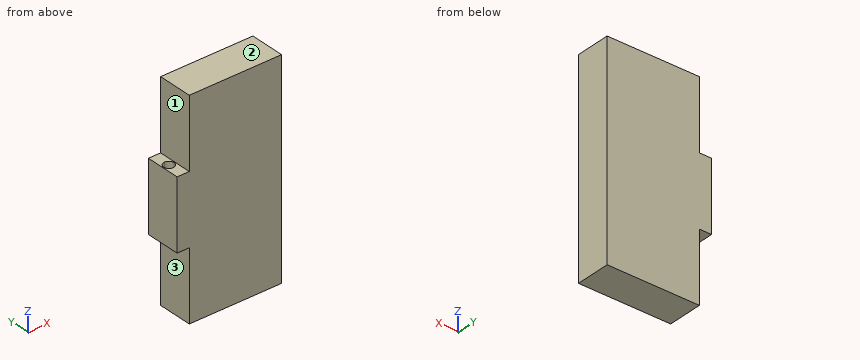
```python
from build123d import *

# Parameters (mm, degrees)
F1_DEPTH = 25.4
F3_DEPTH = 101.601


with BuildPart() as f1:
    # F0 (on Front) → F1 (new body)
    with BuildSketch(Plane.XZ):
        Polygon((0, 25.4), (0, 0), (0, -25.4), (8.89, -25.4), (8.89, -76.2), (76.2, -76.2), (76.2, 76.2), (8.89, 76.2), (8.89, 25.4), align=None)
    extrude(amount=F1_DEPTH)

    # F2 (on face) → F3 (cut, through all)
    with BuildSketch(Plane.XY.offset(25.4)):
        with BuildLine():
            ThreePointArc((8.255, -12.7), (7.139077, -10.005923), (4.445, -8.89))
            ThreePointArc((4.445, -8.89), (1.750923, -15.394077), (8.255, -12.7))
        make_face()
    extrude(amount=-F3_DEPTH, mode=Mode.SUBTRACT)


solid = f1.part
```
Here's how the part is built. I have some questions about the finished solid (model axes, mm). Face numbers are marked on the shaded views. A direction names the side the tool comes from. Coordinates: 2 decimals unless noted, no trailing zeros. Write each loop counter-clockwise with the first axis right and the second up, starting at its lowest first coordinate (ties: lowest second). Pieces come first, ordered by that corner, then holes. Notation, with made-up numbers: (80, 45) -> (94, 45) arc R20 cw to (94, 65) -> close; hole circle Ø6 at (21, 14). An arc over 180 degrees is marked (long way). Use a Markdown table: item, result. Add a question column.
(1) Please list where these lines run through material, in increasing order: line 1 (X direction, y = -15.5, z = 53.5); line 2 (X direction, y = -12.7, z = 9.5) (3 decimals); line 3 (X direction, y = -13.5, z = 23.5).
(2) For the marked faces 1, 2 and 3, which set-ups out of +Z, -Z, +X, -X, +Y, -Y let a thin tool reach every point of the face, with its end or its side?
(3) I'm going to push flat-ended pins straight in: P1, Ø7, axis at x = 3, y = -15, coming from the +Z side; P2, Ø2.5, axis at x = 6.5, y = -17, coming from the -Z side; P3, Ø2, axis at y = -11.5, z = -33.5, coming from the -X side. Where does each tip first touch, or does it pass through?
(4) If we section it at B-B, the plane z = -66: Write out the boundary of the cut face in (x, y).
(5) If we section it at A-A, the plane y = -5.25: Write out the boundary of the cut face in (x, z), and give its area (3 significant figures).
Outcome:
| question | item | result |
|---|---|---|
| 1 | line 1 | x = 8.89 to 76.2 |
| 1 | line 2 | x = 0 to 0.635, 8.255 to 76.2 |
| 1 | line 3 | x = 0 to 0.72, 8.17 to 76.2 |
| 2 | face 1 | +Z, -X, +Y, -Y |
| 2 | face 2 | +Z, +X, -X, +Y, -Y |
| 2 | face 3 | -Z, -X, +Y, -Y |
| 3 | P1 | stops at z = 25.4 |
| 3 | P2 | stops at z = -25.4 |
| 3 | P3 | stops at x = 8.89 |
| 4 | outline | (8.89, -25.4) -> (76.2, -25.4) -> (76.2, 0) -> (8.89, 0) -> close |
| 5 | outline | (0, -25.4) -> (8.89, -25.4) -> (8.89, -76.2) -> (76.2, -76.2) -> (76.2, 76.2) -> (8.89, 76.2) -> (8.89, 25.4) -> (0, 25.4) -> close |
| 5 | area | 10,700 mm^2 |
